Print and shaded views of the part. All mm, measured from the part's lowest x, y and z. Give positions to 0.01 mm unless a question says otherwise; leave off trailing zeros. Loops run counter-clockwise (first coordinate to the right, second up) from the corner with the lowest first, then second, coordinate; pieces in that order, holes last. Notation, with made-up numbers: (80.5, 48.5) - (93.5, 48.5) arc R21 cw to (93.5, 68.5) - close; hole circle Ø1 at (62, 84.25). An arc over 180 degrees is marked (long way). Return JSON: item names as keys, results as strings.
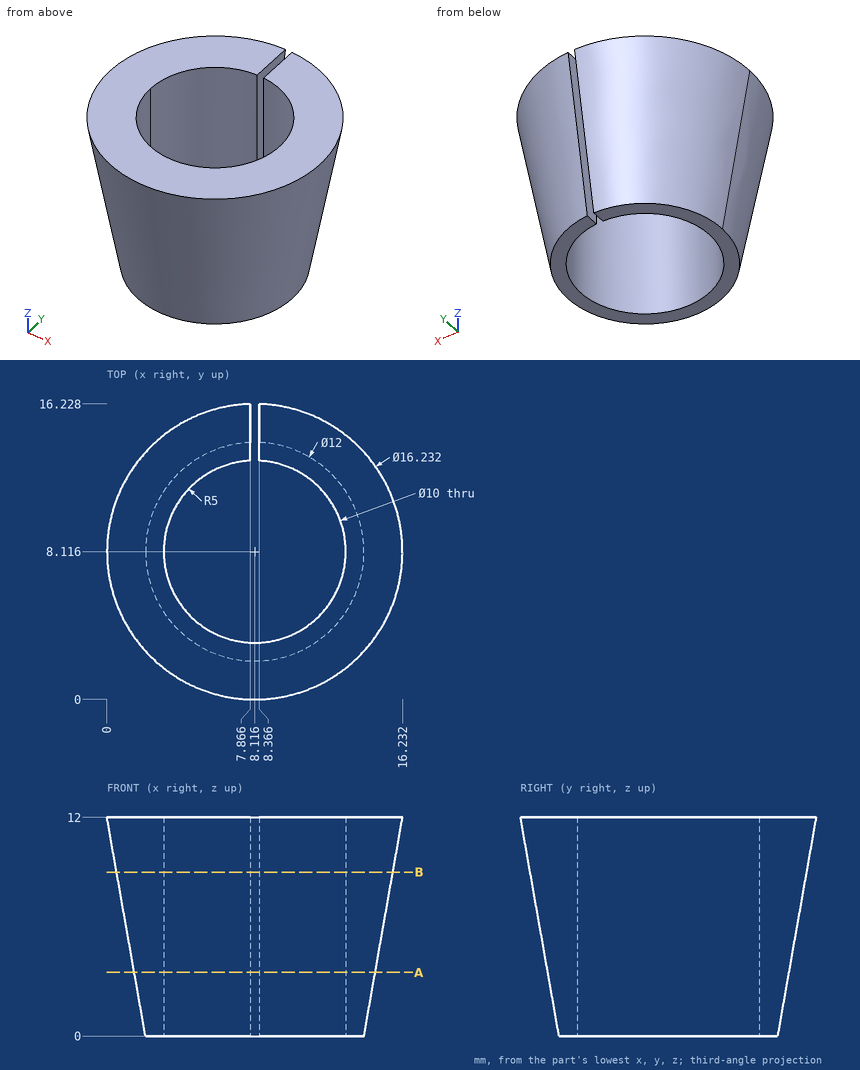
1. Drop flat-ended pins along their axis: P1, Ø1.5, axis at y = 2.5, z = 5.5, coming from the -X side; P2, Ø1.5, axis at y = 9, z = 7, coming from the +X side; P3, Ø3.5, axis at y = 14.5, z = 3.5, coming from the +X side. Give the stop position or say it passes through.
Values follow:
{"P1": "stops at x = 3.1", "P2": "stops at x = 15.45", "P3": "stops at x = 12.89"}
2. Drill centre lines: probe 1 along X at (y, z) = (11.25, 5.5); probe 2 along X at (y, z) = (10.25, 7.5); probe 3 along Y at (x, z) = (10, 6.75) (1 decimal). Where is each one in solid material? Low to high.
Values follow:
{"probe 1": "x = 1.89 to 4.22, 12.01 to 14.34", "probe 2": "x = 1.11 to 3.59, 12.64 to 15.12", "probe 3": "y = 1.2 to 3.5, 12.7 to 15.1"}
3. Cut at B-B, the plane z = 9. Write the cut outline in (x, y).
Values follow:
{"outline": "(7.87, 13.11) - (7.87, 15.7) arc R7.59 ccw (long way) to (8.37, 15.7) - (8.37, 13.11) arc R5 cw (long way) to start"}
4. Cut at A-A, the plane z = 3.5. Write the cut outline in (x, y).
Values follow:
{"outline": "(7.87, 13.11) - (7.87, 14.73) arc R6.62 ccw (long way) to (8.37, 14.73) - (8.37, 13.11) arc R5 cw (long way) to start"}
